from build123d import *

# Parameters (mm, degrees)
F1_DEPTH = 3


with BuildPart() as f1:
    # F0 (on Front) → F1 (new body)
    with BuildSketch(Plane.XZ):
        Polygon((-13.137085, -65.671355), (0, 75.750001), (-7.071068, 68.678933), (-9.192388, 70.800253), (-23.334524, 56.658118), (-21.213203, 54.536797), (-31.819805, 43.930196), (-33.941125, 46.051516), (-48.083261, 31.90938), (-45.961941, 29.78806), (-56.568542, 19.181458), (-58.689863, 21.302779), (-65.760931, 14.231711), (-72.831998, 7.160643), (-70.710678, 5.039323), (-81.31728, -5.567279), (-83.4386, -3.445959), (-97.580736, -17.588094), (-95.459415, -19.709415), (-106.066017, -30.316016), (-108.187338, -28.194696), (-122.329473, -42.336832), (-120.208153, -44.458152), (-127.279221, -51.52922), (-113.137085, -65.671355), (-103.137085, -65.671355), (-103.137085, -68.671355), (-83.137085, -68.671355), (-83.137085, -65.671355), (-73.137085, -65.671355), (-73.137085, -68.671355), (-53.137085, -68.671355), (-53.137085, -65.671355), (-43.137085, -65.671355), (-43.137085, -68.671355), (-23.137085, -68.671355), (-23.137085, -65.671355), align=None)
    extrude(amount=F1_DEPTH)


solid = f1.part
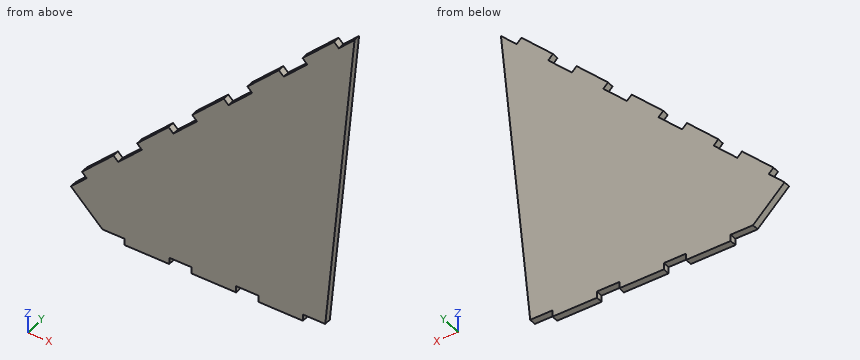
Verification items for the finished model (mm, model axes). Coordinates: 2 decimals unless noted, no trailing zeros. Write each loop counter-clockwise with the first axis right and the second up, starting at its lowest first coordinate (ties: lowest second). Pieces come first, ordered by that corner, then holes. Notation, with made-up numbers: (2, -23.5) -> (15, -23.5) arc R21 ccw to (15, -4.5) -> close; hole circle Ø2 at (30, -38). An arc over 180 degrees is marked (long way). One line per item, written item: value. Start each with the question number.
Q1. Cross-section at B-B on x = -116. Enter the section's corners in (y, z).
Q2. Thickness scan on L1, parallel to X at y = -0.5, z = 69.5; L2, parallel to Z at x = -95, y = -2.5; L3, parallel to Z at x = -112, y = -2.6. Record the ranges inside material, lowest first. Write a range as from..to.
Q3. Go/stop test with flat-tipped pins: P1, Ø0.9, axis at y = -2, z = -67.5, coming from the -X side; P2, Ø1.5, axis at y = -2, z = -7, coming from the -X side; P3, Ø0.9, axis at x = -110.5, y = -2, coming from the -Z side. Record where each tip stops, or that it passes through.
Q4. Cross-section at A-A on z = 2.5. Enter the section's corners in (x, y).
Checked values:
1. outline: (-3, -62.81) -> (0, -62.81) -> (0, -36.01) -> (-3, -36.01) -> close
2. L1: x = -10.49..-7.89, -6.25..-0.58
2. L2: z = -68.67..-15.01
2. L3: z = -65.67..-32.01
3. P1: stops at x = -103.14
3. P2: stops at x = -87.74
3. P3: stops at z = -65.67
4. outline: (-73.25, -3) -> (-6.8, -3) -> (-6.8, 0) -> (-73.25, 0) -> close
